Here's how the part is built. I have some questions about the finished solid (model axes, mm). Round coordinates to 2 decimals unless told otherwise and drop trailing zeros. Loops run counter-clockwise (first coordinate to the right, second up) from the corner with the lowest first, then second, coordinate; pieces in that order, holes last. Notation, with made-up numbers: M 67,77 L 114,77 A9 ccw 114,83 Z; hole C 21.5,-27 d9. An arc over 180 degrees is marked long. Use a Markdown table: item, result.
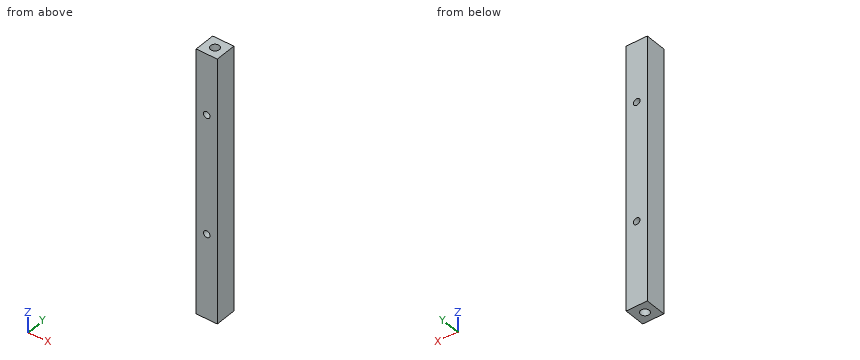
```python
from build123d import *

# Parameters (mm, degrees)
SKETCH1_W                       = 8
SKETCH1_H                       = 8
EXTRUDE1_DEPTH                  = 100
M3_TAPPED_HOLE1_D               = 2.5
M4_TAPPED_HOLE1_D               = 3.3
M4_TAPPED_HOLE1_DEPTH           = 10
M4_TAPPED_HOLE1_TIP             = 0.991420021
M4_TAPPED_HOLE1_ON_FACE_2_D     = 3.3
M4_TAPPED_HOLE1_ON_FACE_2_DEPTH = 10
M4_TAPPED_HOLE1_ON_FACE_2_TIP   = 0.991420021


with BuildPart() as part:
    # Sketch1 → Extrude1 (new body)
    with BuildSketch(Plane.XY):
        with Locations((4, 4)):
            Rectangle(SKETCH1_W, SKETCH1_H)
    extrude(amount=EXTRUDE1_DEPTH)

    # M3 Tapped Hole1 (through all)
    with Locations(Plane(origin=(4, 8, 77), x_dir=(0, 0, 1), z_dir=(0, 1, 0))):
        with Locations((0, 0), (-45, 0)):
            Hole(M3_TAPPED_HOLE1_D / 2)

    # M4 Tapped Hole1
    with Locations(Plane(origin=(4, 4, 0), x_dir=(-1, 0, 0), z_dir=(0, 0, -1))):
        with Locations((0, 0)):
            Hole(M4_TAPPED_HOLE1_D / 2, depth=M4_TAPPED_HOLE1_DEPTH)
            with Locations((0, 0, -(M4_TAPPED_HOLE1_DEPTH + M4_TAPPED_HOLE1_TIP / 2))):  # 118° drill point
                Cone(0, M4_TAPPED_HOLE1_D / 2, M4_TAPPED_HOLE1_TIP, mode=Mode.SUBTRACT)

    # M4 Tapped Hole1 on face 2
    with Locations(Plane(origin=(4, 4, 100), x_dir=(1, 0, 0), z_dir=(0, 0, 1))):
        with Locations((0, 0)):
            Hole(M4_TAPPED_HOLE1_ON_FACE_2_D / 2, depth=M4_TAPPED_HOLE1_ON_FACE_2_DEPTH)
            with Locations((0, 0, -(M4_TAPPED_HOLE1_ON_FACE_2_DEPTH + M4_TAPPED_HOLE1_ON_FACE_2_TIP / 2))):  # 118° drill point
                Cone(0, M4_TAPPED_HOLE1_ON_FACE_2_D / 2, M4_TAPPED_HOLE1_ON_FACE_2_TIP, mode=Mode.SUBTRACT)


solid = part.part
```
Q1. I need wall thicknesses on line 1 (Z direction, x = 3.75, y = 4); line 2 (Z direction, x = 5, y = 7.75); line 3 (X direction, y = 4, z = 95.25). Which ranges of each line are inside material? Lowest first, please. Write a range as from..to.
Return value:
| item | result |
|---|---|
| line 1 | z = 10.84..30.78, 33.22..75.78, 78.22..89.16 |
| line 2 | z = 0..31.25, 32.75..76.25, 77.75..100 |
| line 3 | x = 0..2.35, 5.65..8 |
Q2. Imagine slicing it at A-A, the plane z = 77. Please give me the cut outline in (x, y).
Return value:
| item | result |
|---|---|
| outline | M 0,0 L 2.75,0 L 2.75,8 L 0,8 Z; M 5.25,0 L 8,0 L 8,8 L 5.25,8 Z |
Q3. Will these pins go through, and if not, where does the flat tip stop? P1, Ø2, axis at x = 4, z = 32, coming from the -Y side; P2, Ø3, axis at x = 4, y = 4, coming from the +Z side.
Return value:
| item | result |
|---|---|
| P1 | passes through |
| P2 | stops at z = 89.91 |
